from build123d import *

# Parameters (mm, degrees)
SKETCH1_W           = 74.6
SKETCH1_H           = 62
BOSS_EXTRUDE1_DEPTH = 3.2
CUT_EXTRUDE1_REACH  = 5.2
SKETCH2_W           = 40
SKETCH2_H           = 50
CUT_EXTRUDE2_REACH  = 5.2
SKETCH3_R           = 2.625


with BuildPart() as part:
    # Sketch1 → Boss-Extrude1 (new body)
    with BuildSketch(Plane(origin=(0, 0, 0), x_dir=(0, 0, -1), z_dir=(1, 0, 0))):
        with Locations((37.3, 31)):
            Rectangle(SKETCH1_W, SKETCH1_H)
    extrude(amount=BOSS_EXTRUDE1_DEPTH)

    # Sketch2 → Cut-Extrude1 (cut, up to next)
    with BuildSketch(Plane(origin=(3.2, 0, 0), x_dir=(0, 0, -1), z_dir=(1, 0, 0)), mode=Mode.PRIVATE) as cut_extrude1_sk1:
        with Locations((37.3, 31)):
            Rectangle(SKETCH2_W, SKETCH2_H)
    cut_extrude1_tool1 = extrude(cut_extrude1_sk1.sketch, amount=-CUT_EXTRUDE1_REACH, mode=Mode.PRIVATE) & part.part
    add(cut_extrude1_tool1.solids().sort_by_distance((3.2, 31, -37.3))[0], mode=Mode.SUBTRACT)

    # Sketch3 → Cut-Extrude2 (cut, up to next)
    with BuildSketch(Plane.ZY, mode=Mode.PRIVATE) as cut_extrude2_sk1:
        with Locations((-67.1, 13)):
            Circle(SKETCH3_R)
    cut_extrude2_tool1 = extrude(cut_extrude2_sk1.sketch, amount=-CUT_EXTRUDE2_REACH, mode=Mode.PRIVATE) & part.part
    add(cut_extrude2_tool1.solids().sort_by_distance((0, 13, -67.1))[0], mode=Mode.SUBTRACT)
    # Sketch3 → Cut-Extrude2 (cut, up to next)
    with BuildSketch(Plane.ZY, mode=Mode.PRIVATE) as cut_extrude2_sk2:
        with Locations((-67.1, 49)):
            Circle(SKETCH3_R)
    cut_extrude2_tool2 = extrude(cut_extrude2_sk2.sketch, amount=-CUT_EXTRUDE2_REACH, mode=Mode.PRIVATE) & part.part
    add(cut_extrude2_tool2.solids().sort_by_distance((0, 49, -67.1))[0], mode=Mode.SUBTRACT)
    # Sketch3 → Cut-Extrude2 (cut, up to next)
    with BuildSketch(Plane.ZY, mode=Mode.PRIVATE) as cut_extrude2_sk3:
        with Locations((-7.5, 49)):
            Circle(SKETCH3_R)
    cut_extrude2_tool3 = extrude(cut_extrude2_sk3.sketch, amount=-CUT_EXTRUDE2_REACH, mode=Mode.PRIVATE) & part.part
    add(cut_extrude2_tool3.solids().sort_by_distance((0, 49, -7.5))[0], mode=Mode.SUBTRACT)
    # Sketch3 → Cut-Extrude2 (cut, up to next)
    with BuildSketch(Plane.ZY, mode=Mode.PRIVATE) as cut_extrude2_sk4:
        with Locations((-7.5, 13)):
            Circle(SKETCH3_R)
    cut_extrude2_tool4 = extrude(cut_extrude2_sk4.sketch, amount=-CUT_EXTRUDE2_REACH, mode=Mode.PRIVATE) & part.part
    add(cut_extrude2_tool4.solids().sort_by_distance((0, 13, -7.5))[0], mode=Mode.SUBTRACT)


solid = part.part
Read the model definition and answer for the solid it produces. Units are mm, in the model's axes. A direction names the side the tool comes from. Round coordinates to 2 decimals unless told otherwise and drop trailing zeros. Loops run counter-clockwise (first coordinate to the right, second up) from the corner with the lowest first, then second, coordinate; pieces in that order, holes last.
Q1. Which of the six approach directions +Z, -Z, +X, -X, +Y, -Y give full straight-line access (tool end or side, diameter ignored) to faces 5 (the face through (2, 31, -17.3)), 6 (the face through (2, 31, -74.6))?
Q2. Section C-C on y = 49 is taken. Write down the section's boundary in (x, z) (3 decimals).
Q3. This flat-tipped pin is pushed along its axis until it touches: pin 1 (4.5 mm diameter, centred on y = 49, z = -67.1, fed in from -X). Where does it stop, or does it pass through?
Q4. Section B-B on x = 2.45 is taken. Write down the section's boundary in (y, z) (3 decimals), and give its area (3 significant figures).
Q5. Determine the mould class of faces 1 (the face through (2, 31, 0)), 2 (the face through (2, 31, -57.3)), 3 (the face through (2, 0, -37)), 4 (the face through (1.58, 11.4, -9.58)) for opening direction Y: released by +Y, released by -Y, zero draft, split by the parting line, or undercut.
Q6. Section D-D on z = -33 is taken. Write down the section's boundary in (x, y), and give its area (3 significant figures).
Q7. Consider probe 1 along Y at (x, z) = (1.25, -7.5) (3 decimals); probe 2 along Z at (x, y) = (2.1, 10); probe 3 along Y at (x, z) = (2.15, -46.5). Determine where each line is inside the solid, lowest interval first.
Q8. Section A-A on z = -67.1 is taken. Write down the section's boundary in (x, y) (3 decimals).
Output:
1. face 5: +X, -X
1. face 6: -Z, +X, -X, +Y, -Y
2. outline: (0, -74.6) - (3.2, -74.6) - (3.2, -69.725) - (0, -69.725) - close; (0, -64.475) - (3.2, -64.475) - (3.2, -57.3) - (0, -57.3) - close; (0, -17.3) - (3.2, -17.3) - (3.2, -10.125) - (0, -10.125) - close; (0, -4.875) - (3.2, -4.875) - (3.2, 0) - (0, 0) - close
3. pin 1: passes through
4. outline: (0, -74.6) - (62, -74.6) - (62, 0) - (0, 0) - close; hole (6, -57.3) - (56, -57.3) - (56, -17.3) - (6, -17.3) - close; hole circle Ø5.25 at (13, -67.1); hole circle Ø5.25 at (13, -7.5); hole circle Ø5.25 at (49, -67.1); hole circle Ø5.25 at (49, -7.5)
4. area: 2,540 mm2
5. face 1: zero draft
5. face 2: undercut
5. face 3: released by -Y
5. face 4: undercut
6. outline: (0, 0) - (3.2, 0) - (3.2, 6) - (0, 6) - close; (0, 56) - (3.2, 56) - (3.2, 62) - (0, 62) - close
6. area: 38.4 mm2
7. probe 1: y = 0 to 10.375, 15.625 to 46.375, 51.625 to 62
7. probe 2: z = -74.6 to -57.3, -17.3 to 0
7. probe 3: y = 0 to 6, 56 to 62
8. outline: (0, 0) - (3.2, 0) - (3.2, 10.375) - (0, 10.375) - close; (0, 15.625) - (3.2, 15.625) - (3.2, 46.375) - (0, 46.375) - close; (0, 51.625) - (3.2, 51.625) - (3.2, 62) - (0, 62) - close
